Input: dimensioned drawing with shaded views. Units: mm. Origin: part minimum x, y, z. Give positions to 0.01 mm unless a question says otherwise; leave off trailing zeros. Loops run counter-clockwise (first coordinate to the right, second up) from the corner with the lowest first, then second, coordinate; pieces in that order, holes last.
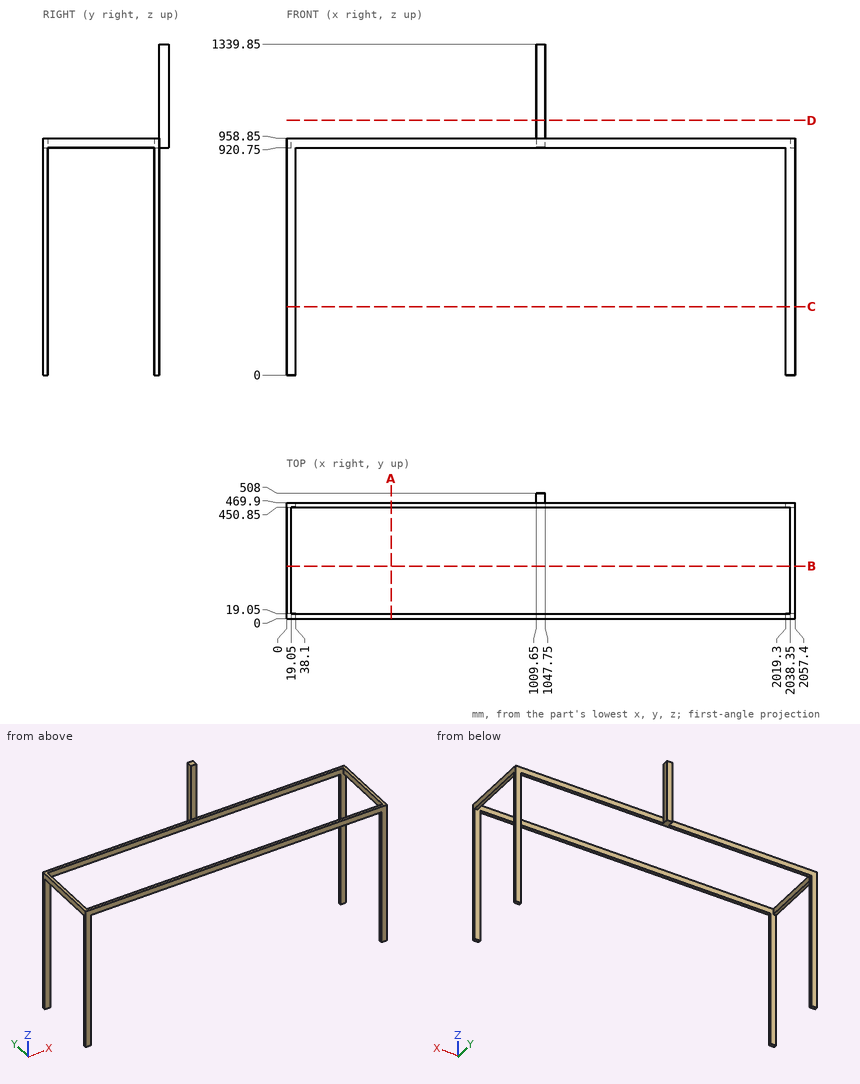
(1) Ray query, line 1 along X through (y, z) = (49.5, 933); line 2 along Z through (x, y) = (225, 460). Return the intervals inside material, ascending.
A:
line 1: x = 0 to 19.05, 2038.35 to 2057.4
line 2: z = 920.75 to 958.85
(2) Section B-B, the plane y = 212.5. Return the cut outline in (x, z).
A:
outline: (0, 920.75) - (19.05, 920.75) - (19.05, 958.85) - (0, 958.85) - close; (2038.35, 920.75) - (2057.4, 920.75) - (2057.4, 958.85) - (2038.35, 958.85) - close
(3) Section D-D, the plane z = 1031. Return the cut outline in (x, y), then the cut area to 3 significant figures.
A:
outline: (1009.65, 469.9) - (1047.75, 469.9) - (1047.75, 508) - (1009.65, 508) - close
area: 1,450 mm2
(4) First-contact query: pin 1 (11.5 mm diameter, centred on y = 131, z = 933.5, fed in from -X); pin 2 (15 mm diameter, centred on x = 2049.5, y = 232, fed in from -Z); pin 3 (19 mm diameter, centred on y = 482.5, z = 1121.5, fed in from +X); pin 4 (19 mm diameter, centred on x = 1037, z = 1080, fed in from -Y). Flat tips, straight axial feed; report the tip coordinate or a pass-through.
A:
pin 1: stops at x = 0
pin 2: stops at z = 920.75
pin 3: stops at x = 1047.75
pin 4: stops at y = 469.9
(5) Section A-A, the plane x = 423.5. Return the cut outline in (y, z), then the cut area to 3 significant figures.
A:
outline: (0, 920.75) - (19.05, 920.75) - (19.05, 958.85) - (0, 958.85) - close; (450.85, 920.75) - (469.9, 920.75) - (469.9, 958.85) - (450.85, 958.85) - close
area: 1,450 mm2
(6) Section C-C, the plane z = 277. Return the cut outline in (x, y).
A:
outline: (0, 0) - (38.1, 0) - (38.1, 19.05) - (0, 19.05) - close; (0, 450.85) - (38.1, 450.85) - (38.1, 469.9) - (0, 469.9) - close; (2019.3, 0) - (2057.4, 0) - (2057.4, 19.05) - (2019.3, 19.05) - close; (2019.3, 450.85) - (2057.4, 450.85) - (2057.4, 469.9) - (2019.3, 469.9) - close
